```python
from build123d import *

# Parameters (mm, degrees)
PAD_DEPTH       = 6.5
POCKET_DEPTH    = 6
SKETCH002_R     = 13.5
POCKET001_DEPTH = 1
SKETCH003_W     = 4.9
SKETCH003_H     = 6.5
PAD001_DEPTH    = 5
POCKET002_DEPTH = 10
SKETCH008_R     = 0.6
POCKET003_DEPTH = 2
SKETCH009_R     = 0.6
POCKET004_DEPTH = 2
FILLET_R        = 3.9
FILLET001_R     = 3.9
FILLET002_R     = 5
FILLET003_R     = 5
FILLET004_R     = 5
FILLET005_R     = 5
SKETCH010_W     = 3.45
SKETCH010_H     = 6.5
PAD002_DEPTH    = 6
POCKET005_DEPTH = 10
SKETCH012_R     = 0.6
POCKET006_DEPTH = 2
SKETCH013_R     = 0.6
POCKET007_DEPTH = 2
FILLET006_R     = 5.9
FILLET007_R     = 5.9


with BuildPart() as part:
    # Sketch → Pad (new body)
    with BuildSketch(Plane.XY):
        with BuildLine():
            Line((-21.862293, 15.5), (-21.862293, -15.5))
            Line((-21.862293, -15.5), (-15.125083, -17.4))
            ThreePointArc((-15.125083, -17.4), (0.226102, -23.053785), (15.463446, -17.1))
            Line((15.463446, -17.1), (22.461838, -16.95))
            Line((22.461838, 16.95), (22.461838, -16.95))
            Line((15.463446, 17.1), (22.461838, 16.95))
            ThreePointArc((15.463446, 17.1), (0.226102, 23.053785), (-15.125083, 17.4))
            Line((-21.862293, 15.5), (-15.125083, 17.4))
        make_face()
    extrude(amount=PAD_DEPTH)

    # Sketch001 → Pocket (cut)
    with BuildSketch(Plane.XY):
        with BuildLine():
            Line((-14.55, 16.55), (-20.805997, 15.2))
            Line((-20.805997, 15.2), (-20.805997, -15.2))
            Line((-20.805997, -15.2), (-14.55, -16.55))
            ThreePointArc((-14.55, -16.55), (0, -22.036447), (14.55, -16.55))
            Line((14.55, -16.55), (21.832857, -16.05))
            Line((21.832857, 16.05), (21.832857, -16.05))
            Line((14.55, 16.55), (21.832857, 16.05))
            ThreePointArc((14.55, 16.55), (0, 22.036447), (-14.55, 16.55))
        make_face()
    extrude(amount=POCKET_DEPTH, mode=Mode.SUBTRACT)

    # Sketch002 (on Face19 of Pocket) → Pocket001 (cut)
    with BuildSketch(Plane(origin=(0, 0, 6), x_dir=(1, 0, 0), z_dir=(0, 0, -1))):
        Circle(SKETCH002_R)
    extrude(amount=-POCKET001_DEPTH, mode=Mode.SUBTRACT)

    # Sketch003 (on Face6 of Pocket001) → Pad001 (join)
    with BuildSketch(Plane.YZ.offset(22.461838)):
        with Locations((-14.5, 3.25)):
            Rectangle(SKETCH003_W, SKETCH003_H)
        with Locations((14.5, 3.25)):
            Rectangle(SKETCH003_W, SKETCH003_H)
    extrude(amount=PAD001_DEPTH)

    # Sketch006 → Pocket002 (cut)
    with BuildSketch(Plane.XY.offset(10)):
        with BuildLine():
            ThreePointArc((22.461838, 16.95), (24.723382, 15.046575), (27.461838, 13.93371))
            Line((27.461838, 16.95), (27.461838, 13.93371))
            Line((27.461838, 16.95), (22.461838, 16.95))
        make_face()
        with BuildLine():
            ThreePointArc((27.461838, -13.93371), (24.723382, -15.046575), (22.461838, -16.95))
            Line((27.461838, -16.95), (22.461838, -16.95))
            Line((27.461838, -13.93371), (27.461838, -16.95))
        make_face()
    extrude(amount=-POCKET002_DEPTH, mode=Mode.SUBTRACT)

    # Sketch008 (on Face27 of Pocket002) → Pocket003 (cut)
    with BuildSketch(Plane(origin=(0, -12.05, 0), x_dir=(-1, 0, 0), z_dir=(0, 1, 0))):
        with Locations((-25.761838, 1.2)):
            Circle(SKETCH008_R)
    extrude(amount=-POCKET003_DEPTH, mode=Mode.SUBTRACT)

    # Sketch009 (on Face26 of Pocket003) → Pocket004 (cut)
    with BuildSketch(Plane.XZ.offset(-12.05)):
        with Locations((25.761838, 1.2)):
            Circle(SKETCH009_R)
    extrude(amount=-POCKET004_DEPTH, mode=Mode.SUBTRACT)

    # Fillet
    fillet_edges = [part.edges().sort_by_distance(p)[0] for p in [
        (27.461838, -12.991855, 6.5),
    ]]
    fillet(fillet_edges, radius=FILLET_R)

    # Fillet001
    fillet001_edges = [part.edges().sort_by_distance(p)[0] for p in [
        (27.461838, 12.991855, 6.5),
    ]]
    fillet(fillet001_edges, radius=FILLET001_R)

    # Fillet002
    fillet002_edges = [part.edges().sort_by_distance(p)[0] for p in [
        (15.463446, -17.1, 3.25),
    ]]
    fillet(fillet002_edges, radius=FILLET002_R)

    # Fillet003
    fillet003_edges = [part.edges().sort_by_distance(p)[0] for p in [
        (15.463446, 17.1, 3.25),
    ]]
    fillet(fillet003_edges, radius=FILLET003_R)

    # Fillet004
    fillet004_edges = [part.edges().sort_by_distance(p)[0] for p in [
        (-15.125083, -17.4, 3.25),
    ]]
    fillet(fillet004_edges, radius=FILLET004_R)

    # Fillet005
    fillet005_edges = [part.edges().sort_by_distance(p)[0] for p in [
        (-15.125083, 17.4, 3.25),
    ]]
    fillet(fillet005_edges, radius=FILLET005_R)

    # Sketch010 (on Face4 of Fillet005) → Pad002 (join)
    with BuildSketch(Plane(origin=(-21.862293, 0, 0), x_dir=(0, -1, 0), z_dir=(-1, 0, 0))):
        with Locations((-13.775, 3.25)):
            Rectangle(SKETCH010_W, SKETCH010_H)
        with Locations((13.775, 3.25)):
            Rectangle(SKETCH010_W, SKETCH010_H)
    extrude(amount=PAD002_DEPTH)

    # Sketch011 (on Face6 of Pad002) → Pocket005 (cut)
    with BuildSketch(Plane.XY.offset(6.5)):
        with BuildLine():
            ThreePointArc((-27.862293, 14.1), (-24.766364, 14.388874), (-21.862293, 15.5))
            Line((-21.862293, 15.5), (-27.862293, 15.5))
            Line((-27.862293, 15.5), (-27.862293, 14.1))
        make_face()
        with BuildLine():
            ThreePointArc((-21.862293, -15.5), (-24.766364, -14.388874), (-27.862293, -14.1))
            Line((-27.862293, -14.1), (-27.862293, -15.5))
            Line((-27.862293, -15.5), (-21.862293, -15.5))
        make_face()
    extrude(amount=-POCKET005_DEPTH, mode=Mode.SUBTRACT)

    # Sketch012 (on Face23 of Pocket005) → Pocket006 (cut)
    with BuildSketch(Plane(origin=(0, -12.05, 0), x_dir=(-1, 0, 0), z_dir=(0, 1, 0))):
        with Locations((26.162293, 1.2)):
            Circle(SKETCH012_R)
    extrude(amount=-POCKET006_DEPTH, mode=Mode.SUBTRACT)

    # Sketch013 (on Face21 of Pocket006) → Pocket007 (cut)
    with BuildSketch(Plane.XZ.offset(-12.05)):
        with Locations((-26.162293, 1.2)):
            Circle(SKETCH013_R)
    extrude(amount=-POCKET007_DEPTH, mode=Mode.SUBTRACT)

    # Fillet006
    fillet006_edges = [part.edges().sort_by_distance(p)[0] for p in [
        (-27.862293, 13.075, 6.5),
    ]]
    fillet(fillet006_edges, radius=FILLET006_R)

    # Fillet007
    fillet007_edges = [part.edges().sort_by_distance(p)[0] for p in [
        (-27.862293, -13.075, 6.5),
    ]]
    fillet(fillet007_edges, radius=FILLET007_R)


solid = part.part
```
Model file for the job. Use its own axes, mm. A direction names the side the tool comes from. Give positions to 0.01 mm unless a question says otherwise; leave off trailing zeros. Loops run counter-clockwise (first coordinate to the right, second up) from the corner with the lowest first, then second, coordinate; pieces in that order, holes last. Notation, with made-up numbers: (-10.75, 85.25) -> (39.25, 85.25) arc R22 cw to (39.25, 94.25) -> close; hole circle Ø9 at (3, 86.5). An arc over 180 degrees is marked (long way). Write each question's results on one line, items separated by ' | '.
(1) Cut at A-A on x = 0. List the corners of the cut face in (y, z).
Geometry results:
outline: (-23.05, 0) -> (-22.04, 0) -> (-22.04, 6) -> (-13.5, 6) -> (-13.5, 6.5) -> (-23.05, 6.5) -> close; (13.5, 6) -> (22.04, 6) -> (22.04, 0) -> (23.05, 0) -> (23.05, 6.5) -> (13.5, 6.5) -> close
(2) Probe line 1 along Y through (x, z) = (0, 6.1); line 2 along X through (y, z) = (3.5, 4); line 3 along Y through (x, z) = (-14.5, 3.25). List the from-to ranges inside material, lowest first.
Geometry results:
line 1: y = -23.05 to -13.5, 13.5 to 23.05 | line 2: x = -21.86 to -20.81, 21.83 to 22.46 | line 3: y = -17.93 to -16.59, 16.59 to 17.93
(3) Cut at B-B on y = 0. List the corners of the cut face in (x, z).
Geometry results:
outline: (-21.86, 0) -> (-20.81, 0) -> (-20.81, 6) -> (-13.5, 6) -> (-13.5, 6.5) -> (-21.86, 6.5) -> close; (13.5, 6) -> (21.83, 6) -> (21.83, 0) -> (22.46, 0) -> (22.46, 6.5) -> (13.5, 6.5) -> close
(4) Tool access for faces 4 (the cylindrical face through (-0.222, -22.035, 2.958)), 5 (the flat face through (-24, -12.05, 2)), 6 (the cylindrical face through (-26.084, -13.036, 1.795)), 7 (the cylindrical face through (-15.23, 17.47, 3.3)): list every direction of +Z, -Z, +X, -X, +Y, -Y with a clear straight run to the whole face (end or side of a thin tool).
Geometry results:
face 4: -Z | face 5: +Z, -Z, -X | face 6: none | face 7: +Z, -Z, -X, +Y
(5) Flat gauge pins, fed straight in: pin 1 Ø2 at (x, z) = (-2.5, 4) entering from -Y; pin 2 Ø3 at (y, z) = (-7, 1) entering from -X; pin 3 Ø1.6 at (x, z) = (-26.16, 1.2) entering from +Y. Where does each tip first touch, or does it go through?
Geometry results:
pin 1: stops at y = -23.01 | pin 2: stops at x = -21.86 | pin 3: stops at y = 14.27
(6) Pull direction Z, two halves, no side cores. Call faces 1 (the flat face through (18.14, -16.304, 2.958)), 2 (the cylindrical face through (25.208, -13.036, 0.97)), 3 (the flat face through (10, 10, 6)): released by +Z, released by -Z, zero draft, split by the parting line, or undercut.
Geometry results:
face 1: zero draft | face 2: undercut | face 3: released by -Z
(7) Cut at D-D on x = 16. List the corners of the cut face in (y, z), and give its area (3 significant figures).
Geometry results:
outline: (-17.24, 0) -> (-16.45, 0) -> (-16.45, 6) -> (16.45, 6) -> (16.45, 0) -> (17.24, 0) -> (17.24, 6.5) -> (-17.24, 6.5) -> close | area: 26.7 mm²
